Build history of the part. All positions in model axes, mm. Round coordinates to 2 decimals unless told otherwise and drop trailing zeros. Loops run counter-clockwise (first coordinate to the right, second up) from the corner with the lowest first, then second, coordinate; pieces in that order, holes last.
from build123d import *

# Parameters (mm, degrees)
IZIM1_R                     = 1
Y_KSEKLIK_EKSTR_ZYON1_DEPTH = 1
RADYUS1_R                   = 2
RADYUS2_R                   = 0.5


with BuildPart() as part:
    # Çizim1 → Yükseklik-Ekstrüzyon1 (new body)
    with BuildSketch(Plane.XY):
        with BuildLine():
            Line((-2, -5.562315087), (-2, -10.562315087))
            ThreePointArc((-2, -10.562315087), (0, 10.75), (2, -10.562315087))
            Line((2, -10.562315087), (2, -5.562315087))
            Line((2, -5.562315087), (5.956773529, -5.562315087))
            ThreePointArc((5.956773529, -5.562315087), (0, 8.15), (-5.956773529, -5.562315087))
            Line((-5.956773529, -5.562315087), (-2, -5.562315087))
        make_face()
        with Locations((-3.5, -8.15)):
            Circle(IZIM1_R, mode=Mode.SUBTRACT)
        with Locations((3.5, -8.15)):
            Circle(IZIM1_R, mode=Mode.SUBTRACT)
    extrude(amount=Y_KSEKLIK_EKSTR_ZYON1_DEPTH)

    # Radyus1
    radyus1_edges = [part.edges().sort_by_distance(p)[0] for p in [
        (-2, -5.562315087, 0.5),
        (2, -5.562315087, 0.5),
        (5.956773529, -5.562315087, 0.5),
        (-5.956773529, -5.562315087, 0.5),
    ]]
    fillet(radyus1_edges, radius=RADYUS1_R)

    # Radyus2
    radyus2_edges = [part.edges().sort_by_distance(p)[0] for p in [
        (-2, -10.562315087, 0.5),
        (2, -10.562315087, 0.5),
    ]]
    fillet(radyus2_edges, radius=RADYUS2_R)


solid = part.part
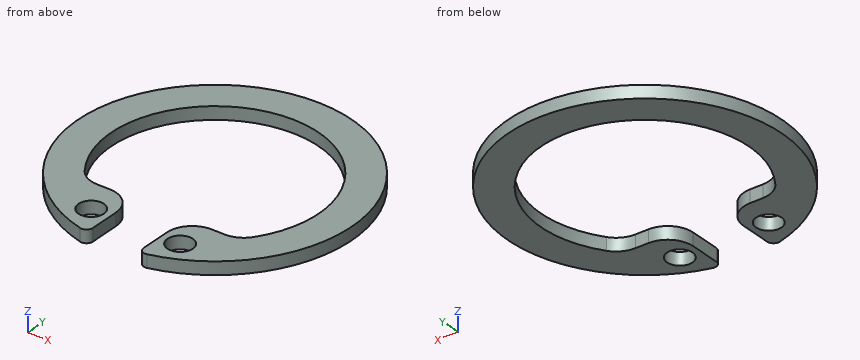
(1) Slice it at C-C on y = -3. List the corners of the cut face in (x, z).
Responses:
outline: (-10.32, 0) - (-7.58, 0) - (-7.58, 1) - (-10.32, 1) - close; (7.58, 0) - (10.32, 0) - (10.32, 1) - (7.58, 1) - close
(2) Pin check, flat tip, straight feed: P1, Ø0.5, axis at y = -8, z = 0.5, coming from the +X side. Stop position of the tip, or through.
Responses:
P1: stops at x = 7.45
(3) Slice it at B-B on x = -3. List the corners of the cut face in (y, z), plus the area to 3 significant figures.
Responses:
outline: (-10.32, 0) - (-9.02, 0) - (-9.02, 1) - (-10.32, 1) - close; (-7.28, 0) - (-5.83, 0) - (-5.83, 1) - (-7.28, 1) - close; (7.58, 0) - (10.32, 0) - (10.32, 1) - (7.58, 1) - close
area: 5.51 mm2
(4) Slice it at D-D on z = 0.65. List the corners of the cut face in (x, y).
Responses:
outline: (-6.64, -4.72) arc R8.15 cw (long way) to (6.64, -4.72) arc R2 cw to (5.01, -5.56) - (4, -5.56) arc R2 ccw to (2, -7.56) - (2, -9.94) arc R0.5 ccw to (2.62, -10.43) arc R10.75 ccw (long way) to (-2.62, -10.43) arc R0.5 ccw to (-2, -9.94) - (-2, -7.56) arc R2 ccw to (-4, -5.56) - (-5.01, -5.56) arc R2 cw to start; hole circle Ø2 at (-3.5, -8.15); hole circle Ø2 at (3.5, -8.15)
(5) Slice it at A-A on y = -8.15. List the corners of the cut face in (x, z), plus the area to 3 significant figures.
Responses:
outline: (-7.01, 0) - (-4.5, 0) - (-4.5, 1) - (-7.01, 1) - close; (-2.5, 0) - (-2, 0) - (-2, 1) - (-2.5, 1) - close; (2, 0) - (2.5, 0) - (2.5, 1) - (2, 1) - close; (4.5, 0) - (7.01, 0) - (7.01, 1) - (4.5, 1) - close
area: 6.02 mm2
(6) Probe line 1 (Y direction, x = -3.25, z = 0.3); line 2 (X direction, y = 0, z = 0.4); line 3 (Y direction, x = -3.5, z = 0.2). List the from-to ranges inside material, lowest first.
Responses:
line 1: y = -10.25 to -9.12, -7.18 to -5.71, 7.47 to 10.25
line 2: x = -10.75 to -8.15, 8.15 to 10.75
line 3: y = -10.16 to -9.15, -7.15 to -5.63, 7.36 to 10.16
